Part model, mm, in its own coordinate system. A direction names the side the tool comes from. Give positions to 0.01 mm unless a question says otherwise; leave off trailing zeros. Order: outer loops, then holes, each group sorted by start corner. A loop starts at its lowest first (then second) coordinate and runs counter-clockwise, first axis right, second up. Notation, with made-up numbers: (77.5, -11.5) -> (88.5, -11.5) arc R13 ccw to (88.5, -0.5) -> close; hole circle Ø6 at (12.5, 24.5). An arc over 180 degrees is marked (long way). Write item = value, one per line. Start each with the question number.
(1) Saw through at D-D, the plane z = 10.75. List the corners of the cut face in (x, y).
(2) Saw through at C-C, the plane x = -17.75. List the corners of the cut face in (y, z) (1 decimal), then the cut area to 3 significant figures.
(3) Saw through at B-B, the plane z = 3.75. List the corners of the cut face in (x, y), then the cut area to 3 significant figures.
(4) Which spindle directions (+Z, -Z, +X, -X, +Y, -Y) get a long thin tool onto all of the face, cutting with end or side? Do faces 1 (the flat face through (-10, 0, 0)), 2 (the cylindrical face through (-12.64, -14.61, 5.55)). Say none if no direction does.
(5) Probe line 1 along Y through (x, z) = (-13.75, 7.5); line 2 along Y through (x, z) = (-3, 11); line 3 along Y through (x, z) = (-11.5, 11.75). List the from-to ranges inside material, lowest first. Write a range as from..to.
(6) Two-plate mould, pull along Y, no slides. Class faces 3 (the flat face through (-10, 32.5, 8)), 4 (the cylindrical face through (-12.64, 10.39, 5.55)), 5 (the flat face through (-10, -32.5, 8)): pulls with the +Y half, pulls with the -Y half, needs draft (parallel to the pull), parting line crosses it, or undercut.
(7) Saw through at A-A, the plane y = -25. List the corners of the cut face in (x, z), then the cut area to 3 significant figures.
Autodesk Inventor part; units mm, degrees
ref_plane "YZ Plane" through (0, 0, 0) normal (1, 0, 0) x (0, 1, 0)
ref_plane "XZ Plane" through (0, 0, 0) normal (0, 1, 0) x (-1, 0, 0)
ref_plane "XY Plane" through (0, 0, 0) normal (0, 0, 1) x (1, 0, 0)
sketch "Sketch1" plane through (0, 0, 0) normal (0, 1, 0) x (-1, 0, 0)
  line L0 (0, 0) -> (20.3, 0)
  line L1 (20.3, 0) -> (20.3, 15)
  line L2 (20.3, 15) -> (0, 15)
  line L3 (0, 15) -> (0, 0)
  dimension "d0" = 15
  dimension "d1" = 20.3
extrude "Extrusion1" add sketch "Sketch1" along normal mid plane 65
sketch "Sketch2" plane through (-20.3, -32.5, 15) normal (-1, 0, 0) x (0, 0, 1)
  circle A0 centre (-7.5, 7.5) radius 3.25
  circle A1 centre (-7.5, 57.5) radius 3.25
  circle A2 centre (-7.5, 7.5) radius 5.5
  circle A3 centre (-7.5, 57.5) radius 5.5
  line L0 (0, 0) -> (-15, 0)
  line L1 (-15, 32.5) -> (12.3047, 32.5) construction
  dimension "d4" = 6.5
  dimension "d5" = 6.5
  dimension "d8" = 11
  dimension "d9" = 11
  dimension "d26" = 25
  dimension "d27" = 25
extrude "Extrusion2" cut sketch "Sketch2" against normal through all contours A0 | A1
extrude "Extrusion3" cut sketch "Sketch2" against normal blind 21.3
sketch "Sketch3" plane through (-20.3, -32.5, 15) normal (-1, 0, 0) x (0, 0, 1)
  circle A0 centre (-7.5, 16.395) radius 3
  line L0 (0, 0) -> (-15, 0)
  circle A1 centre (-7.5, 41.395) radius 3
  point P0 (-15, 32.5)
  dimension "d14" = 6
  dimension "d22" = 16.395
  dimension "d23" = 6
  dimension "d24" = 25
hole "Hole1" at (-20.3, -16.105, 7.5) at (-20.3, 8.895, 7.5) direction (1, 0, 0) diameter 4.917 depth 15.1 tip angle 118
sketch "Sketch4" plane through (-20.3, -32.5, 15) normal (-1, 0, 0) x (0, 0, 1)
  point P0 (-15, 32.5)
properties part number "HeadbarHolderBracket_v2" material "Aluminum 6061"
Results list:
q1.outline = (-20.3, -32.5) -> (0, -32.5) -> (0, -29.44) -> (-20.3, -29.44) -> close; (-20.3, -20.56) -> (0, -20.56) -> (0, 20.56) -> (-20.3, 20.56) -> close; (-20.3, 29.44) -> (0, 29.44) -> (0, 32.5) -> (-20.3, 32.5) -> close
q2.outline = (-32.5, 0) -> (32.5, 0) -> (32.5, 15) -> (-32.5, 15) -> close; hole circle Ø11 at (-25, 7.5); hole circle Ø4.9 at (-16.1, 7.5); hole circle Ø4.9 at (8.9, 7.5); hole circle Ø11 at (25, 7.5)
q2.area = 747 mm^2
q3.outline = (-20.3, -32.5) -> (0, -32.5) -> (0, -29.02) -> (-20.3, -29.02) -> close; (-20.3, -20.98) -> (0, -20.98) -> (0, 20.98) -> (-20.3, 20.98) -> close; (-20.3, 29.02) -> (0, 29.02) -> (0, 32.5) -> (-20.3, 32.5) -> close
q3.area = 993 mm^2
q4.face_1 = -Z, +X, -X, +Y, -Y
q4.face_2 = -X
q5.line_1 = -32.5..-30.5, -19.5..-18.56, -13.65..6.44, 11.35..19.5, 30.5..32.5
q5.line_2 = -32.5..-29.24, -20.76..20.76, 29.24..32.5
q5.line_3 = -32.5..-28.49, -21.51..21.51, 28.49..32.5
q6.face_3 = pulls with the +Y half
q6.face_4 = undercut
q6.face_5 = pulls with the -Y half
q7.outline = (-20.3, 0) -> (0, 0) -> (0, 2) -> (-20.3, 2) -> close; (-20.3, 13) -> (0, 13) -> (0, 15) -> (-20.3, 15) -> close
q7.area = 81.2 mm^2
